Study the drawing (mm; zero at the part's minimum x, y, z) and answer. Round coordinates to 2 decimals unless told otherwise and drop trailing zeros. Order: outer loops, then holes, each group sorted by start corner. A loop starts at its lowest first (then second) coordinate and runs counter-clockwise, first axis right, second up. Notation, with made-up numbers: (60.5, -15.75) - (76.5, -15.75) arc R25 cw to (76.5, 1.25) - close; hole circle Ø3 at (15, -8.5). An arc over 180 degrees is marked (long way). Put each result on its own line as item: value. Start each with the question number.
Q1. Section D-D on z = 2.1 is taken. Give the vertices of the cut face in (x, y).
Q2. Find the intervals of material crossed by line 1 along Y through (x, z) = (60, 1.65); line 2 along Y through (x, z) = (25, 1.1), in increasing order. Write a range as from..to.
Q3. Section A-A on y = 110 is taken. Give the vertices of the cut face in (x, z), then the cut area to 3 significant figures.
Q4. Section B-B on x = 60 is taken. Give the vertices of the cut face in (y, z), then the cut area to 3 significant figures.
Q5. Section C-C on y = 92 is taken. Give the vertices of the cut face in (x, z).
Q6. This flat-tipped pin is pushed along its axis until it touches: pin 1 Ø5 at (x, y) = (20, 110) entering from +Z. Where does it stop, or does it pass through?
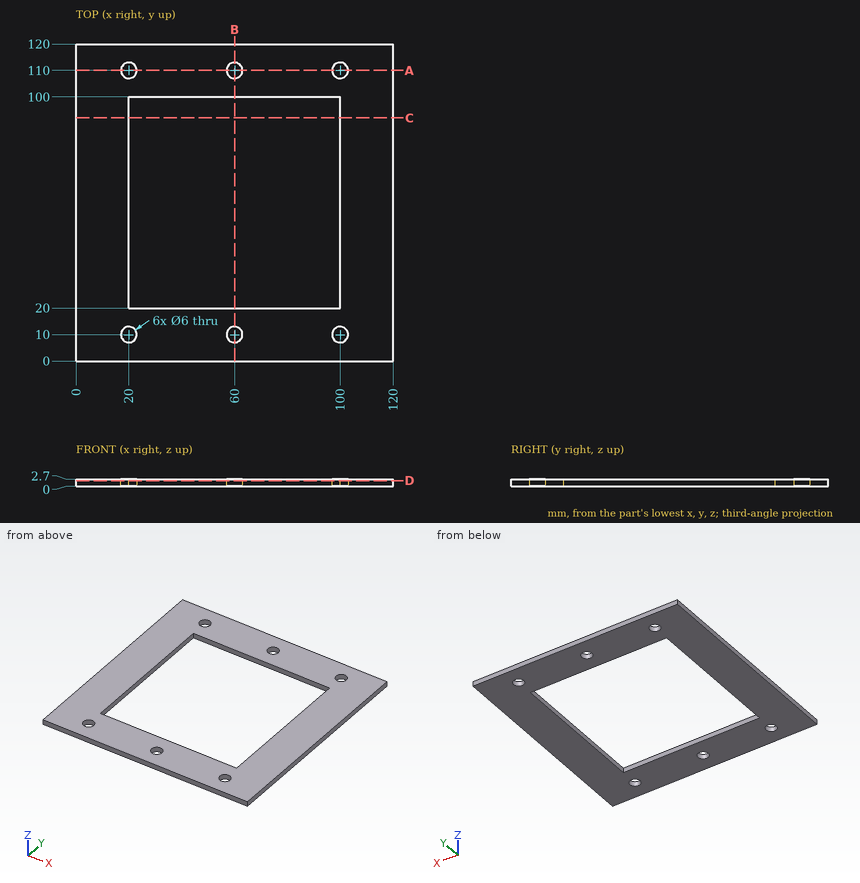
Findings:
1. outline: (0, 0) - (120, 0) - (120, 120) - (0, 120) - close; hole circle Ø6 at (20, 10); hole circle Ø6 at (20, 110); hole (20, 20) - (100, 20) - (100, 100) - (20, 100) - close; hole circle Ø6 at (60, 10); hole circle Ø6 at (60, 110); hole circle Ø6 at (100, 10); hole circle Ø6 at (100, 110)
2. line 1: 0..7, 13..20, 100..107, 113..120
2. line 2: 0..20, 100..120
3. outline: (0, 0) - (17, 0) - (17, 2.7) - (0, 2.7) - close; (23, 0) - (57, 0) - (57, 2.7) - (23, 2.7) - close; (63, 0) - (97, 0) - (97, 2.7) - (63, 2.7) - close; (103, 0) - (120, 0) - (120, 2.7) - (103, 2.7) - close
3. area: 275 mm2
4. outline: (0, 0) - (7, 0) - (7, 2.7) - (0, 2.7) - close; (13, 0) - (20, 0) - (20, 2.7) - (13, 2.7) - close; (100, 0) - (107, 0) - (107, 2.7) - (100, 2.7) - close; (113, 0) - (120, 0) - (120, 2.7) - (113, 2.7) - close
4. area: 75.6 mm2
5. outline: (0, 0) - (20, 0) - (20, 2.7) - (0, 2.7) - close; (100, 0) - (120, 0) - (120, 2.7) - (100, 2.7) - close
6. pin 1: through
